Read the model definition and answer for the solid it produces. Units are mm, in the model's axes. A direction names the side the tool comes from. Round coordinates to 2 decimals unless told otherwise and drop trailing zeros. Loops run counter-clockwise (first coordinate to the right, second up) from the corner with the lowest first, then second, coordinate; pieces in that order, holes last. Notation, with made-up numbers: (36.25, 82) - (59.25, 82) arc R14 ccw to (59.25, 103) - close; hole circle Ø10 at (-10, 49.25). An arc over 180 degrees is marked (long way). Use one line per item in the form item = value. Start each with the question number.
```python
from build123d import *

# Parameters (mm, degrees)
F0_R     = 1.5
F1_DEPTH = 2


with BuildPart() as f1:
    # F0 (on Top) → F1 (new body)
    with BuildSketch(Plane.XY):
        with BuildLine():
            ThreePointArc((0, 5), (1.4644660941, 1.4644660941), (5, 0))
            Line((5, 0), (95, 0))
            ThreePointArc((95, 0), (98.5355339059, 1.4644660941), (100, 5))
            Line((100, 5), (100, 35))
            ThreePointArc((100, 35), (98.5355339059, 38.5355339059), (95, 40))
            Line((95, 40), (5, 40))
            ThreePointArc((5, 40), (1.4644660941, 38.5355339059), (0, 35))
            Line((0, 35), (0, 5))
        make_face()
        Polygon((21.7325409239, 5), (8.3096175434, 5), (8.3096175434, 29.0790486555), (11.1080361987, 29.0790486555), (11.1080361987, 7.5349140738), (21.7325409239, 7.5349140738), align=None, mode=Mode.SUBTRACT)
        with BuildLine():
            Line((25.2108013994, 23.0500638312), (27.9775995049, 23.0500638312))
            Line((27.9775995049, 23.0500638312), (27.9775995049, 11.3399202304))
            add(Edge.make_bspline(
                [(27.9775995049, 11.3399202304), (27.9775995049, 9.1317518376), (28.9815519603, 8.0461129619)],
                knots=[0, 0, 0, 1, 1, 1], degree=2))
            add(Edge.make_bspline(
                [(28.9815519603, 8.0461129619), (29.9855044157, 6.9604740862), (32.1251616173, 6.9604740862)],
                knots=[0, 0, 0, 1, 1, 1], degree=2))
            add(Edge.make_bspline(
                [(32.1251616173, 6.9604740862), (34.960470914, 6.9604740862), (36.2674536382, 8.5072459795)],
                knots=[0, 0, 0, 1, 1, 1], degree=2))
            add(Edge.make_bspline(
                [(36.2674536382, 8.5072459795), (37.5744363623, 10.0540178727), (37.5744363623, 13.563898898)],
                knots=[0, 0, 0, 1, 1, 1], degree=2))
            Line((37.5744363623, 13.563898898), (37.5744363623, 23.0500638312))
            Line((37.5744363623, 23.0500638312), (40.3096139181, 23.0500638312))
            Line((40.3096139181, 23.0500638312), (40.3096139181, 5))
            Line((40.3096139181, 5), (38.0540147006, 5))
            Line((38.0540147006, 5), (37.6587578284, 7.418972058))
            Line((37.6587578284, 7.418972058), (37.5111952628, 7.418972058))
            add(Edge.make_bspline(
                [(37.5111952628, 7.418972058), (36.6732506937, 6.0856388757), (35.1818147625, 5.3768115515)],
                knots=[0, 0, 0, 1, 1, 1], degree=2))
            add(Edge.make_bspline(
                [(35.1818147625, 5.3768115515), (33.6903788313, 4.6679842273), (31.7773355698, 4.6679842273)],
                knots=[0, 0, 0, 1, 1, 1], degree=2))
            add(Edge.make_bspline(
                [(31.7773355698, 4.6679842273), (28.4835283013, 4.6679842273), (26.8471648503, 6.2332014413)],
                knots=[0, 0, 0, 1, 1, 1], degree=2))
            add(Edge.make_bspline(
                [(26.8471648503, 6.2332014413), (25.2108013994, 7.7984186553), (25.2108013994, 11.2397884894)],
                knots=[0, 0, 0, 1, 1, 1], degree=2))
            Line((25.2108013994, 11.2397884894), (25.2108013994, 23.0500638312))
        make_face(mode=Mode.SUBTRACT)
        with BuildLine():
            add(Edge.make_bspline(
                [(57.880099411, 5.611330629), (56.0724579821, 4.6679842273), (53.3214701514, 4.6679842273)],
                knots=[0, 0, 0, 1, 1, 1], degree=2))
            add(Edge.make_bspline(
                [(53.3214701514, 4.6679842273), (49.400521979, 4.6679842273), (47.2503245942, 7.0816861937)],
                knots=[0, 0, 0, 1, 1, 1], degree=2))
            add(Edge.make_bspline(
                [(47.2503245942, 7.0816861937), (45.1001272093, 9.49538816), (45.1001272093, 13.9117249456)],
                knots=[0, 0, 0, 1, 1, 1], degree=2))
            add(Edge.make_bspline(
                [(45.1001272093, 13.9117249456), (45.1001272093, 18.4387336554), (47.2845801898, 20.9104066296)],
                knots=[0, 0, 0, 1, 1, 1], degree=2))
            add(Edge.make_bspline(
                [(47.2845801898, 20.9104066296), (49.4690331702, 23.3820796039), (53.5006532668, 23.3820796039)],
                knots=[0, 0, 0, 1, 1, 1], degree=2))
            add(Edge.make_bspline(
                [(53.5006532668, 23.3820796039), (54.8023658993, 23.3820796039), (56.1040785318, 23.1001297017)],
                knots=[0, 0, 0, 1, 1, 1], degree=2))
            add(Edge.make_bspline(
                [(56.1040785318, 23.1001297017), (57.4057911643, 22.8181797995), (58.1436039925, 22.4387332022)],
                knots=[0, 0, 0, 1, 1, 1], degree=2))
            Line((58.1436039925, 22.4387332022), (57.3056594234, 20.1198928852))
            add(Edge.make_bspline(
                [(57.3056594234, 20.1198928852), (56.3992036631, 20.4835292076), (55.3293750623, 20.720683331)],
                knots=[0, 0, 0, 1, 1, 1], degree=2))
            add(Edge.make_bspline(
                [(55.3293750623, 20.720683331), (54.2595464615, 20.9578374543), (53.4374121673, 20.9578374543)],
                knots=[0, 0, 0, 1, 1, 1], degree=2))
            add(Edge.make_bspline(
                [(53.4374121673, 20.9578374543), (47.935436506, 20.9578374543), (47.935436506, 13.9433454954)],
                knots=[0, 0, 0, 1, 1, 1], degree=2))
            add(Edge.make_bspline(
                [(47.935436506, 13.9433454954), (47.935436506, 10.6179176771), (49.2766748257, 8.8392617521)],
                knots=[0, 0, 0, 1, 1, 1], degree=2))
            add(Edge.make_bspline(
                [(49.2766748257, 8.8392617521), (50.6179131455, 7.0606058272), (53.2529589602, 7.0606058272)],
                knots=[0, 0, 0, 1, 1, 1], degree=2))
            add(Edge.make_bspline(
                [(53.2529589602, 7.0606058272), (55.5085581777, 7.0606058272), (57.880099411, 8.030302687)],
                knots=[0, 0, 0, 1, 1, 1], degree=2))
            Line((57.880099411, 8.030302687), (57.880099411, 5.611330629))
        make_face(mode=Mode.SUBTRACT)
        with BuildLine():
            Line((75.2924821551, 5), (73.2634968777, 5))
            Line((73.2634968777, 5), (72.7206774398, 7.5718047152))
            Line((72.7206774398, 7.5718047152), (72.5889251491, 7.5718047152))
            add(Edge.make_bspline(
                [(72.5889251491, 7.5718047152), (71.2397816919, 5.8748352105), (69.8985433722, 5.2714097189)],
                knots=[0, 0, 0, 1, 1, 1], degree=2))
            add(Edge.make_bspline(
                [(69.8985433722, 5.2714097189), (68.5573050525, 4.6679842273), (66.54413005, 4.6679842273)],
                knots=[0, 0, 0, 1, 1, 1], degree=2))
            add(Edge.make_bspline(
                [(66.54413005, 4.6679842273), (63.8616534106, 4.6679842273), (62.3385969296, 6.0540183259)],
                knots=[0, 0, 0, 1, 1, 1], degree=2))
            add(Edge.make_bspline(
                [(62.3385969296, 6.0540183259), (60.8155404487, 7.4400524245), (60.8155404487, 9.9907767732)],
                knots=[0, 0, 0, 1, 1, 1], degree=2))
            add(Edge.make_bspline(
                [(60.8155404487, 9.9907767732), (60.8155404487, 15.455861793), (69.5586224621, 15.7193663745)],
                knots=[0, 0, 0, 1, 1, 1], degree=2))
            Line((69.5586224621, 15.7193663745), (72.6205456989, 15.8194981155))
            Line((72.6205456989, 15.8194981155), (72.6205456989, 16.9420276326))
            add(Edge.make_bspline(
                [(72.6205456989, 16.9420276326), (72.6205456989, 19.0658745593), (71.708819847, 20.0777321522)],
                knots=[0, 0, 0, 1, 1, 1], degree=2))
            add(Edge.make_bspline(
                [(71.708819847, 20.0777321522), (70.7970939951, 21.089589745), (68.7839189926, 21.089589745)],
                knots=[0, 0, 0, 1, 1, 1], degree=2))
            add(Edge.make_bspline(
                [(68.7839189926, 21.089589745), (66.5283197751, 21.089589745), (63.6824702951, 19.7088257381)],
                knots=[0, 0, 0, 1, 1, 1], degree=2))
            Line((63.6824702951, 19.7088257381), (62.8392556344, 21.801052115))
            add(Edge.make_bspline(
                [(62.8392556344, 21.801052115), (64.1725888167, 22.5230546683), (65.761521443, 22.9341218154)],
                knots=[0, 0, 0, 1, 1, 1], degree=2))
            add(Edge.make_bspline(
                [(65.761521443, 22.9341218154), (67.3504540693, 23.3451889625), (68.9525619247, 23.3451889625)],
                knots=[0, 0, 0, 1, 1, 1], degree=2))
            add(Edge.make_bspline(
                [(68.9525619247, 23.3451889625), (72.177858002, 23.3451889625), (73.7351700785, 21.9143590851)],
                knots=[0, 0, 0, 1, 1, 1], degree=2))
            add(Edge.make_bspline(
                [(73.7351700785, 21.9143590851), (75.2924821551, 20.4835292076), (75.2924821551, 17.3214742299)],
                knots=[0, 0, 0, 1, 1, 1], degree=2))
            Line((75.2924821551, 17.3214742299), (75.2924821551, 5))
        make_face(mode=Mode.SUBTRACT)
        with BuildLine():
            add(Edge.make_bspline(
                [(91.4347728164, 12.9051374443), (92.5625724251, 11.7193668277), (92.5625724251, 9.922265582)],
                knots=[0, 0, 0, 1, 1, 1], degree=2))
            add(Edge.make_bspline(
                [(92.5625724251, 9.922265582), (92.5625724251, 7.4031617831), (90.686419805, 6.0355730052)],
                knots=[0, 0, 0, 1, 1, 1], degree=2))
            add(Edge.make_bspline(
                [(90.686419805, 6.0355730052), (88.8102671849, 4.6679842273), (85.4163281755, 4.6679842273)],
                knots=[0, 0, 0, 1, 1, 1], degree=2))
            add(Edge.make_bspline(
                [(85.4163281755, 4.6679842273), (81.8273957757, 4.6679842273), (79.8194908649, 5.8063240193)],
                knots=[0, 0, 0, 1, 1, 1], degree=2))
            Line((79.8194908649, 5.8063240193), (79.8194908649, 8.3412380931))
            add(Edge.make_bspline(
                [(79.8194908649, 8.3412380931), (81.1212034974, 7.6824766394), (82.6100043827, 7.3056650879)],
                knots=[0, 0, 0, 1, 1, 1], degree=2))
            add(Edge.make_bspline(
                [(82.6100043827, 7.3056650879), (84.0988052681, 6.9288535364), (85.4848393666, 6.9288535364)],
                knots=[0, 0, 0, 1, 1, 1], degree=2))
            add(Edge.make_bspline(
                [(85.4848393666, 6.9288535364), (87.6244965682, 6.9288535364), (88.7760115893, 7.6113304024)],
                knots=[0, 0, 0, 1, 1, 1], degree=2))
            add(Edge.make_bspline(
                [(88.7760115893, 7.6113304024), (89.9275266104, 8.2938072685), (89.9275266104, 9.6956516419)],
                knots=[0, 0, 0, 1, 1, 1], degree=2))
            add(Edge.make_bspline(
                [(89.9275266104, 9.6956516419), (89.9275266104, 10.7496699678), (89.0158007584, 11.4980229792)],
                knots=[0, 0, 0, 1, 1, 1], degree=2))
            add(Edge.make_bspline(
                [(89.0158007584, 11.4980229792), (88.1040749065, 12.2463759906), (85.4479487252, 13.2687737668)],
                knots=[0, 0, 0, 1, 1, 1], degree=2))
            add(Edge.make_bspline(
                [(85.4479487252, 13.2687737668), (82.9288449263, 14.2068500768), (81.8669214629, 14.9077722636)],
                knots=[0, 0, 0, 1, 1, 1], degree=2))
            add(Edge.make_bspline(
                [(81.8669214629, 14.9077722636), (80.8049979996, 15.6086944503), (80.2858939741, 16.4967048899)],
                knots=[0, 0, 0, 1, 1, 1], degree=2))
            add(Edge.make_bspline(
                [(80.2858939741, 16.4967048899), (79.7667899486, 17.3847153295), (79.7667899486, 18.6179167708)],
                knots=[0, 0, 0, 1, 1, 1], degree=2))
            add(Edge.make_bspline(
                [(79.7667899486, 18.6179167708), (79.7667899486, 20.8260851636), (81.5638911942, 22.1040823837)],
                knots=[0, 0, 0, 1, 1, 1], degree=2))
            add(Edge.make_bspline(
                [(81.5638911942, 22.1040823837), (83.3609924399, 23.3820796039), (86.4861567763, 23.3820796039)],
                knots=[0, 0, 0, 1, 1, 1], degree=2))
            add(Edge.make_bspline(
                [(86.4861567763, 23.3820796039), (89.4005174474, 23.3820796039), (92.1883959194, 22.1963089873)],
                knots=[0, 0, 0, 1, 1, 1], degree=2))
            Line((92.1883959194, 22.1963089873), (91.213428968, 19.9723303196))
            add(Edge.make_bspline(
                [(91.213428968, 19.9723303196), (88.4993317787, 21.089589745), (86.291163386, 21.089589745)],
                knots=[0, 0, 0, 1, 1, 1], degree=2))
            add(Edge.make_bspline(
                [(86.291163386, 21.089589745), (84.3464995747, 21.089589745), (83.3583573941, 20.4808941618)],
                knots=[0, 0, 0, 1, 1, 1], degree=2))
            add(Edge.make_bspline(
                [(83.3583573941, 20.4808941618), (82.3702152136, 19.8721985786), (82.3702152136, 18.8023699778)],
                knots=[0, 0, 0, 1, 1, 1], degree=2))
            add(Edge.make_bspline(
                [(82.3702152136, 18.8023699778), (82.3702152136, 18.0750973329), (82.7417566735, 17.5665334907)],
                knots=[0, 0, 0, 1, 1, 1], degree=2))
            add(Edge.make_bspline(
                [(82.7417566735, 17.5665334907), (83.1132981333, 17.0579696484), (83.9354324275, 16.5968366308)],
                knots=[0, 0, 0, 1, 1, 1], degree=2))
            add(Edge.make_bspline(
                [(83.9354324275, 16.5968366308), (84.7575667218, 16.1357036133), (87.0974874053, 15.2608684028)],
                knots=[0, 0, 0, 1, 1, 1], degree=2))
            add(Edge.make_bspline(
                [(87.0974874053, 15.2608684028), (90.3069732077, 14.090908061), (91.4347728164, 12.9051374443)],
                knots=[0, 0, 0, 1, 1, 1], degree=2))
        make_face(mode=Mode.SUBTRACT)
        with Locations((5, 35)):
            Circle(F0_R, mode=Mode.SUBTRACT)
    extrude(amount=F1_DEPTH)


solid = f1.part
```
1) A cutting plane is placed at B-B on y = 27. Write down the section's boundary in (x, z), plus the area to 3 significant figures.
2) Determine the mould class of faces 1 (the cylindrical face through (1, 2, 1)), 2 (the flat face through (11.108, 18, 1)), 3 (the flat face through (49, 25, 0)) for opening direction X: +X half, -X half, draft (parallel to the pull), parting line (faces both ways), or undercut.
3) For faces 4 (the flat face through (25.211, 17, 1)), 5 (the flat face through (51, 40, 1)), determine the directions among +Z, -Z, +X, -X, +Y, -Y from which every point of the face is accessible in a straight line to the end or side of a thin tool.
4) A cutting plane is placed at C-C on z = 1.2. Count the separate pieces of the cut face and the enclosed holes in it, plus the area to 3 significant figures.
5) A cutting plane is placed at A-A on x = 16.5. Write down the section's boundary in (y, z).
6) Straight lines are drawn through the part: line 1 (X direction, y = 27, z = 1.6); line 2 (Y direction, x = 32, z = 1.7); line 3 (Y direction, x = 5, z = 0.65). For each, find the intervals that lie inside material, in ascending order. Write a range as from..to.
Checks:
q1.outline = (0, 0) - (8.31, 0) - (8.31, 2) - (0, 2) - close; (11.11, 0) - (100, 0) - (100, 2) - (11.11, 2) - close
q1.area = 194 mm²
q2.face_1 = -X half
q2.face_2 = undercut
q2.face_3 = draft
q3.face_4 = +Z, -Z
q3.face_5 = +Z, -Z, +X, -X, +Y
q4.separate_pieces = 1
q4.enclosed_holes = 6
q4.area = 3,390 mm²
q5.outline = (0, 0) - (5, 0) - (5, 2) - (0, 2) - close; (7.53, 0) - (40, 0) - (40, 2) - (7.53, 2) - close
q6.line_1 = 0..8.31, 11.11..100
q6.line_2 = 0..4.67, 6.96..40
q6.line_3 = 0..33.5, 36.5..40
